Check sheet for the modelled part. Datum: model origin and axes. Units: mm. Give positions to 0.01 mm unless a question says otherwise; leave off trailing zeros. Loops run counter-clockwise (first coordinate to the right, second up) from the corner with the lowest first, then second, coordinate; pieces in that order, holes last. Notation, with made-up numbers: (-33, 71.25) - (-17, 71.25) arc R27 cw to (-17, 98.25) - close; hole circle Ø5 at (80.25, 62.25). An arc over 180 degrees is marked (long way). Answer in a Markdown table with one row per item. Add a question column.
(1) Sectioned sample at B-B on z = 1. Enter the section's corners in (x, y), then the cut area to 3 significant figures.
(2) Thickness scan on L1, parallel to Y at x = 0, z = 0; L2, parallel to Y at x = 0, z = -6; L3, parallel to X at y = 1, z = -6. Record the ranges inside material, lowest first.
(3) Go/stop test with flat-tipped pins: P1, Ø6, axis at x = -1, z = -6.5, coming from the -Y side; P2, Ø5, axis at x = -5, y = -7, coming from the +Z side (3 decimals); P3, Ø8, axis at y = 5, z = 4, coming from the -X side; P4, Ø4, axis at x = 0, y = 0, coming from the -Z side. Record where each tip stops, or that it passes through.
(4) Sectioned sample at A-A on z = -1.5. Enter the section's corners in (x, y).
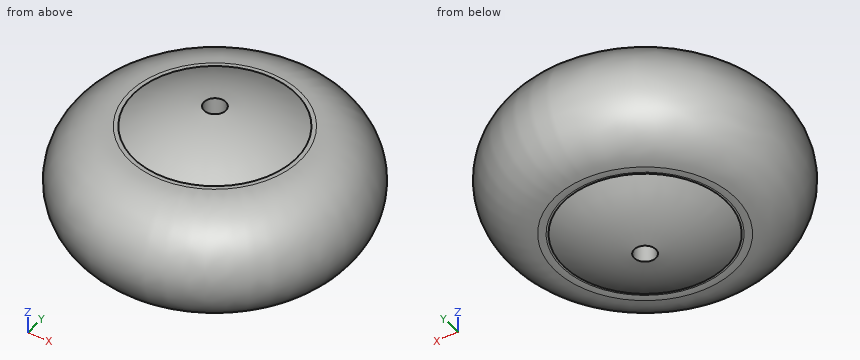
from build123d import *

# Parameters (mm, degrees)
F2_R          = 1.5
F3_DEPTH      = 10.9897371298
F3_DEPTH_BACK = 10.99934016


with BuildPart() as f1:
    # F0 (on Front) → F1 (revolve)
    with BuildSketch(Plane.XZ):
        with BuildLine():
            Line((-11.5125622961, -7.9851364725), (-11.2310720272, -7.9852245345))
            ThreePointArc((-11.2310720272, -7.9852245345), (-5.8128750802, -10.2248932597), (0, -10.9887371298))
            Line((0, -10.9887371298), (0, 10.99834016))
            ThreePointArc((0, 10.99834016), (-5.8099761259, 10.2352713467), (-11.2258712218, 7.997822597))
            Line((-11.2258712218, 7.997822597), (-11.8122072176, 7.9977955632))
            ThreePointArc((-11.8122072176, 7.9977955632), (-19.9927642859, 0.3401750584), (-12.4924337781, -7.9848299277))
            Line((-12.4924337781, -7.9848299277), (-11.5125622961, -7.9851364725))
        make_face()
        with BuildLine():
            ThreePointArc((-12.4924337781, -7.9848299277), (-12.0025027349, -7.9999996085), (-11.5125622961, -7.9851364725))
            Line((-11.5125622961, -7.9851364725), (-12.4924337781, -7.9848299277))
        make_face()
    revolve(axis=Axis((0, 0, 0.0048015151), (0, 0, -1)))

    # F2 (on Top) → F3 (cut, two sides)
    with BuildSketch(Plane.XY) as f3_sk:
        Circle(F2_R)
    extrude(amount=-F3_DEPTH, mode=Mode.SUBTRACT)
    extrude(f3_sk.sketch, amount=F3_DEPTH_BACK, mode=Mode.SUBTRACT)


solid = f1.part
Reply:
| question | item | result |
|---|---|---|
| 1 | outline | circle Ø39.87 at (0, 0); hole circle Ø3 at (0, 0) |
| 1 | area | 1,240 mm^2 |
| 2 | L1 | -20 to -1.5, 1.5 to 20 |
| 2 | L2 | -17.29 to -1.5, 1.5 to 17.29 |
| 2 | L3 | -17.26 to -1.12, 1.12 to 17.26 |
| 3 | P1 | y = -19.17 |
| 3 | P2 | z = 10.155 |
| 3 | P3 | x = -19.8 |
| 3 | P4 | z = -10.94 |
| 4 | outline | circle Ø39.72 at (0, 0); hole circle Ø3 at (0, 0) |
